Geometry: final body of the model. Coordinates: model frame, mm. Face numbers are marked on the shaded views. A direction names the side the tool comes from. Round coordinates to 2 decimals unless told otherwise and drop trailing zeros. Loops run counter-clockwise (first coordinate to the right, second up) from the corner with the lowest first, then second, coordinate; pieces in that order, holes last. Notation, with made-up numbers: (17.5, 40) - (53.5, 40) arc R5 cw to (53.5, 49) - close; hole circle Ø6 at (59.5, 84). An arc over 180 degrees is marked (long way). Answer as a JSON object with one key per item and string values. Group by question number.
Item 1: Section D-D (x = -15). Return the cut outline in (y, z), plus the area to 3 significant figures.
Item 2: First-contact query: pin 1 (8 mm diameter, centred on x = 15, y = 16, fed in from +Z); pin 2 (16 mm diameter, centred on x = -0.5, z = -5.5, fed in from +Y); pin 3 (6 mm diameter, centred on x = 12, y = 6.5, fed in from -Z). Flat tips, straight axial feed; report the tip coordinate or a pass-through.
Item 3: Draft query along Z for the marked faces 1, 2, 3 and 4. Return one class per face: released by +Z, released by -Z, zero draft, split by the parting line, or undercut.
Item 4: Section B-B (z = 0). Return the cut outline in (x, y).
Item 5: Section A-A (x = 0). Return the cut outline in (y, z).
Item 6: Reachability of the marked faces 5 and 6 from +Z, -Z, +X, -X, +Y, -Y: full face, straight path, thin tool, end or side. Return the list, or none.
Item 7: Section C-C (y = 7). Return the cut outline in (x, z).
Item 8: Line query: line 1 (Z direction, x = 0, y = 21); line 2 (Z direction, x = 0, y = 5.5); line 3 (X direction, y = 19.25, z = 7.5). Output: solid intervals per line, ascending.
Autodesk Inventor part; units mm, degrees
ref_plane "YZ Plane" through (0, 0, 0) normal (1, 0, 0) x (0, 1, 0)
ref_plane "XZ Plane" through (0, 0, 0) normal (0, 1, 0) x (-1, 0, 0)
ref_plane "XY Plane" through (0, 0, 0) normal (0, 0, 1) x (1, 0, 0)
sketch "Sketch1" plane through (0, 0, 0) normal (0, 1, 0) x (-1, 0, 0)
  circle A0 centre (0, 0) radius 19
  dimension "d0" = 38
extrude "Extrusion1" add sketch "Sketch1" along normal blind 25.4
sketch "Sketch3" plane through (0, 0, 0) normal (0, -1, 0) x (1, 0, 0)
  circle A0 centre (0, 0) radius 19
  circle A1 centre (0, 0) radius 16
  dimension "d9" = 32
extrude "Extrusion3" cut sketch "Sketch3" against normal blind 5
thread "Thread2"
sketch "Sketch4" plane through (0, 25.4, 0) normal (0, 1, 0) x (1, 0, 0)
  circle A0 centre (0, 0) radius 16
  dimension "d14" = 32
extrude "Extrusion4" cut sketch "Sketch4" against normal blind 17.78
thread "Thread3"
sketch "Sketch5" plane through (0, 0, 0) normal (0, -1, 0) x (1, 0, 0)
  circle A0 centre (0, 0) radius 12.5
  dimension "d19" = 25
extrude "Extrusion5" cut sketch "Sketch5" against normal blind 17.78
properties part number "NA1-1PiezoExtension"
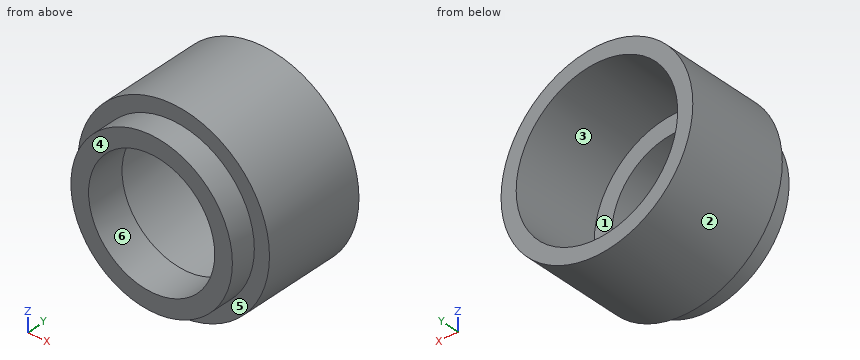
Values:
{
 "1": {"outline": "(0, -5.57) - (5, -5.57) - (5, -11.66) - (25.4, -11.66) - (25.4, -5.57) - (7.62, -5.57) - (7.62, 5.57) - (25.4, 5.57) - (25.4, 11.66) - (5, 11.66) - (5, 5.57) - (0, 5.57) - close", "area": "333 mm^2"},
 "2": {"pin 1": "stops at z = 15.49", "pin 2": "stops at y = 7.62", "pin 3": "stops at z = -16.73"},
 "3": {"face 1": "undercut", "face 2": "split by the parting line", "face 3": "undercut", "face 4": "zero draft"},
 "4": {"outline": "(-19, 5) - (-16, 5) - (-16, 0) - (-12.5, 0) - (-12.5, 7.62) - (-16, 7.62) - (-16, 25.4) - (-19, 25.4) - close; (12.5, 0) - (16, 0) - (16, 5) - (19, 5) - (19, 25.4) - (16, 25.4) - (16, 7.62) - (12.5, 7.62) - close"},
 "5": {"outline": "(0, -16) - (5, -16) - (5, -19) - (25.4, -19) - (25.4, -16) - (7.62, -16) - (7.62, -12.5) - (0, -12.5) - close; (0, 12.5) - (7.62, 12.5) - (7.62, 16) - (25.4, 16) - (25.4, 19) - (5, 19) - (5, 16) - (0, 16) - close"},
 "6": {"face 5": "-Y", "face 6": "+Y, -Y"},
 "7": {"outline": "circle Ø38 at (0, 0); hole circle Ø25 at (0, 0)"},
 "8": {"line 1": "z = -19 to -16, 16 to 19", "line 2": "z = -19 to -12.5, 12.5 to 19", "line 3": "x = -17.46 to -14.13, 14.13 to 17.46"}
}
